from build123d import *

# Parameters (mm, degrees)
SKETCH1_R               = 6.25
BOSS_EXTRUDE1_DEPTH     = 32.5
SKETCH2_R               = 3.75
CUT_EXTRUDE1_DEPTH      = 11.000075787
CUT_EXTRUDE1_DEPTH_BACK = 25.999924213
CUT_EXTRUDE2_REACH      = 71.956
SKETCH3_R               = 6.25
CHAMFER1_SIZE           = 10


with BuildPart() as part:
    # Sketch1 → Boss-Extrude1 (new body)
    with BuildSketch(Plane.XY):
        with BuildLine():
            Line((0, 12.5), (-32.5, 12.5))
            Line((-32.5, 12.5), (-32.5, 5))
            Line((-32.5, 5), (-11.456439237, 5))
            ThreePointArc((-11.456439237, 5), (-10.470155046, -6.828312626), (-0.043527687, -12.499924213))
            Line((-0.043527687, -12.499924213), (37.456472313, -12.499924213))
            Line((37.456472313, -12.499924213), (37.456472313, 22.500075787))
            Line((37.456472313, 22.500075787), (29.956472313, 22.500075787))
            Line((29.956472313, 22.500075787), (29.956472313, -4.999924213))
            Line((29.956472313, -4.999924213), (11.456472313, -4.999924213))
            ThreePointArc((11.456472313, -4.999924213), (10.458227686, 6.84656656), (0, 12.5))
        make_face()
        Circle(SKETCH1_R, mode=Mode.SUBTRACT)
    extrude(amount=BOSS_EXTRUDE1_DEPTH)

    # Sketch2 → Cut-Extrude1 (cut, two sides)
    with BuildSketch(Plane(origin=(0, 12.5, 0), x_dir=(1, 0, 0), z_dir=(0, 1, 0))) as cut_extrude1_sk:
        with Locations((-22.5, -7.5)):
            Circle(SKETCH2_R)
        with Locations((-22.5, -25)):
            Circle(SKETCH2_R)
    extrude(amount=CUT_EXTRUDE1_DEPTH, mode=Mode.SUBTRACT)
    extrude(cut_extrude1_sk.sketch, amount=-CUT_EXTRUDE1_DEPTH_BACK, mode=Mode.SUBTRACT)

    # Sketch3 → Cut-Extrude2 (cut, up to next)
    with BuildSketch(Plane(origin=(37.456472313, 0, 0), x_dir=(0, 0, -1), z_dir=(1, 0, 0)), mode=Mode.PRIVATE) as cut_extrude2_sk1:
        with Locations((-16.3, 7.500075787)):
            Circle(SKETCH3_R)
    cut_extrude2_tool1 = extrude(cut_extrude2_sk1.sketch, amount=-CUT_EXTRUDE2_REACH, mode=Mode.PRIVATE) & part.part
    add(cut_extrude2_tool1.solids().sort_by_distance((37.456472, 7.500076, 16.3))[0], mode=Mode.SUBTRACT)

    # Chamfer1
    chamfer1_edges = [part.edges().sort_by_distance(p)[0] for p in [
        (33.706472313, 22.500075787, 0),
        (33.706472313, 22.500075787, 32.5),
    ]]
    chamfer(chamfer1_edges, length=CHAMFER1_SIZE)


solid = part.part
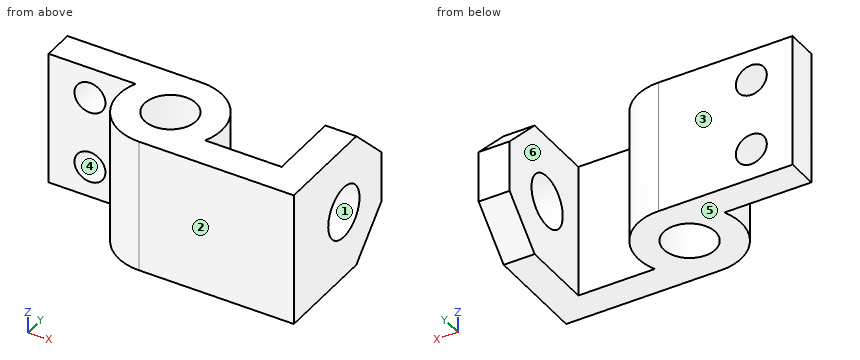
Read the model definition and answer for the solid it produces. Units are mm, in the model's axes. Face numbers are marked on the shaded views. A direction names the side the tool comes from. Give positions to 0.01 mm unless a question says otherwise; leave off trailing zeros. Write each loop counter-clockwise with the first axis right and the second up, starting at its lowest first coordinate (ties: lowest second). Pieces come first, ordered by that corner, then holes. Notation, with made-up numbers: (6.25, 18) - (41.25, 18) arc R16 cw to (41.25, 28) - close; hole circle Ø9 at (61, 16). An arc over 180 degrees is marked (long way). Answer in a Markdown table with one row per item. Add a question column.
Item 1: Determine the mould class of the marked faces 4, 5 and 6 for opening direction Z: pulls with the +Z half, pulls with the -Z half, needs draft (parallel to the pull), parting line crosses it, or undercut.
Item 2: Section C-C, the plane x = -25 is taken. Write down the section's boundary in (y, z), and give its area (3 significant figures).
Item 3: Flat-ended cylindrical pins translate along their axes: P1, Ø6, axis at x = 0, z = 21.5, coming from the +Y side; P2, Ø8, axis at y = 19, z = 8.5, coming from the -X side; P3, Ø10, axis at x = 0, y = 0, coming from the +Z side; P4, Ø4, axis at x = 3.5, z = 7.5, coming from the +Y side. Find the tip coordinate at first contact, or state that the pin passes through.
Item 4: Section D-D, the plane y = 10.5 is taken. Write down the section's boundary in (x, z), and give its area (3 significant figures).
Item 5: Section B-B, the plane y = 0 is taken. Write down the section's boundary in (x, z).
Item 6: Section A-A, the plane z = 16.3 is taken. Write down the section's boundary in (x, y).
Item 7: A tool of negligible diameter and unlimited length cuts with its end or side. For the marked faces 1, 2 and 3, from which of +Z, -Z, +X, -X, +Y, -Y can it reach the whole face along a straight path? Write none if from no direction.
Item 8: Find the intervals of material crossed by L1, parallel to Z at x = -22.5, y = 7; L2, parallel to Y at x = 0, z = 15.5; L3, parallel to X at y = 10.75, z = 7.5, in increasing order.
Recorded:
| question | item | result |
|---|---|---|
| 1 | face 4 | undercut |
| 1 | face 5 | pulls with the -Z half |
| 1 | face 6 | needs draft |
| 2 | outline | (5, 0) - (12.5, 0) - (12.5, 4.7) - (5, 4.7) - close; (5, 10.3) - (12.5, 10.3) - (12.5, 22.2) - (5, 22.2) - close; (5, 27.8) - (12.5, 27.8) - (12.5, 32.5) - (5, 32.5) - close |
| 2 | area | 160 mm2 |
| 3 | P1 | stops at y = 12.5 |
| 3 | P2 | stops at x = 29.96 |
| 3 | P3 | passes through |
| 3 | P4 | stops at y = 12.41 |
| 4 | outline | (-32.5, 0) - (6.78, 0) - (6.78, 32.5) - (-32.5, 32.5) - close; (29.96, 0) - (37.46, 0) - (37.46, 10.82) - (29.96, 10.82) - close; (29.96, 21.78) - (37.46, 21.78) - (37.46, 32.5) - (29.96, 32.5) - close; hole circle Ø7.5 at (-22.5, 7.5); hole circle Ø7.5 at (-22.5, 25) |
| 4 | area | 1,350 mm2 |
| 5 | outline | (-12.5, 0) - (-6.25, 0) - (-6.25, 32.5) - (-12.5, 32.5) - close; (6.25, 0) - (12.5, 0) - (12.5, 32.5) - (6.25, 32.5) - close; (29.96, 0) - (37.46, 0) - (37.46, 32.5) - (29.96, 32.5) - close |
| 6 | outline | (-32.5, 5) - (-11.46, 5) arc R12.5 ccw to (-0.04, -12.5) - (37.46, -12.5) - (37.46, 1.25) - (29.96, 1.25) - (29.96, -5) - (11.46, -5) arc R12.5 ccw to (0, 12.5) - (-32.5, 12.5) - close; (29.96, 13.75) - (37.46, 13.75) - (37.46, 22.5) - (29.96, 22.5) - close; hole circle Ø12.5 at (0, 0) |
| 7 | face 1 | +X |
| 7 | face 2 | +Z, -Z, +X, -X, -Y |
| 7 | face 3 | +Z, -Z, -X, +Y |
| 8 | L1 | z = 0 to 3.75, 11.25 to 21.25, 28.75 to 32.5 |
| 8 | L2 | y = -12.5 to -6.25, 6.25 to 12.5 |
| 8 | L3 | x = -32.5 to -26.25, -18.75 to 6.38, 29.96 to 37.46 |
